```python
from build123d import *

# Parameters (mm, degrees)
SKETCH_1_R          = 7
EXTRUDE_1_DEPTH     = 25
CUT_EXTRUDE_START   = 25
SKETCH_2_R          = 2.5
CUT_EXTRUDE_1_DEPTH = 10
SKETCH_3_R          = 4
CUT_EXTRUDE_2_DEPTH = 15
FILLET_1_R          = 0.25
CHAMFER_1_SIZE      = 0.3


with BuildPart() as part:
    # 草图1 → 凸台-拉伸1 (new body)
    with BuildSketch(Plane(origin=(0, 0, 0), x_dir=(1, 0, 0), z_dir=(0, 1, 0))):
        with Locations(Location((0, 0, 0), (0, 0, 270))):
            Circle(SKETCH_1_R)
    extrude(amount=EXTRUDE_1_DEPTH)

    # 草图2 → 切除-拉伸1 (cut)
    with BuildSketch(Plane(origin=(0, 0, 0), x_dir=(1, 0, 0), z_dir=(0, 1, 0)).offset(CUT_EXTRUDE_START)):
        with Locations(Location((0, 0, 0), (0, 0, 270))):
            Circle(SKETCH_2_R)
    extrude(amount=-CUT_EXTRUDE_1_DEPTH, mode=Mode.SUBTRACT)

    # 草图3 → 切除-拉伸2 (cut)
    with BuildSketch(Plane(origin=(0, 0, 0), x_dir=(1, 0, 0), z_dir=(0, 1, 0))):
        with Locations(Location((0, 0, 0), (0, 0, 270))):
            Circle(SKETCH_3_R)
    extrude(amount=CUT_EXTRUDE_2_DEPTH, mode=Mode.SUBTRACT)

    # 圆角1
    fillet_1_edges = [part.edges().sort_by_distance(p)[0] for p in [
        (0, 0, -7),
        (0, 25, -7),
    ]]
    fillet(fillet_1_edges, radius=FILLET_1_R)

    # 倒角1
    chamfer_1_edges = [part.edges().sort_by_distance(p)[0] for p in [
        (0, 0, -4),
        (0, 25, -2.5),
    ]]
    chamfer(chamfer_1_edges, length=CHAMFER_1_SIZE)


solid = part.part
```
Part model, mm, in its own coordinate system. A direction names the side the tool comes from. Coordinates: 2 decimals unless noted, no trailing zeros. Loops run counter-clockwise (first coordinate to the right, second up) from the corner with the lowest first, then second, coordinate; pieces in that order, holes last. Notation, with made-up numbers: (-19, 8) - (-14, 8) arc R7 cw to (-14, 15) - close; hole circle Ø8 at (-5, 46.25). An arc over 180 degrees is marked (long way). Write item = value, one per line. Start each with the question number.
Item 1: Cut at A-A, the plane z = 0. Give the cut face in (x, y), and give its area (3 significant figures).
Item 2: Cut at B-B, the plane x = 0. Give the cut face in (y, z), and give its area (3 significant figures).
Item 3: Mould opens along X. For faces 1 (the cylindrical face through (-6.834, 12.328, -1.517)), 2 (the flat face through (-1.4, 0, 4.4)), 3 (the cylindrical face through (-3.905, 7.547, -0.867)) say: released by +X, released by -X, zero draft, split by the parting line, or undercut.
Item 4: Cut at D-D, the plane y = 21.75. Give the cut face in (x, z), and give its area (3 significant figures).
Item 5: Wall check: L1, parallel to X at y = 8.25, z = 0; L2, parallel to X at y = 18, z = 0; L3, parallel to Z at x = -0.75, y = 8.75. Give the ranges that are in metal, low to high. Write a range as from..to.
Item 6: Flat gauge pins, fed straight in: pin 1 Ø1 at (x, z) = (3, -5.5) entering from -Y; pin 2 Ø3 at (y, z) = (11, -5) entering from -X; pin 3 Ø2 at (x, y) = (2, 20) entering from -Z; pin 4 Ø4.5 at (x, z) = (0, 0) entering from -Y. Where does each tip first touch, or does it go through?
Item 7: 3-axis set-ups, long thin cutter, end or side, ignore diameter. For faces 4 (the flat face through (2, 15, 2)), 5 (the flat face through (0, 25, 3)): which of +Z, -Z, +X, -X, +Y, -Y reach the whole face in a straight line?
Item 8: Cut at C-C, the plane y = 4.25. Give the cut face in (x, z).
The answers:
q1.outline = (-7, 0.25) arc R0.25 ccw to (-6.75, 0) - (-4.3, 0) - (-4, 0.3) - (-4, 15) - (-2.5, 15) - (-2.5, 24.7) - (-2.8, 25) - (-6.75, 25) arc R0.25 ccw to (-7, 24.75) - close; (2.5, 15) - (4, 15) - (4, 0.3) - (4.3, 0) - (6.75, 0) arc R0.25 ccw to (7, 0.25) - (7, 24.75) arc R0.25 ccw to (6.75, 25) - (2.8, 25) - (2.5, 24.7) - close
q1.area = 180 mm2
q2.outline = (0, -6.75) arc R0.25 ccw to (0.25, -7) - (24.75, -7) arc R0.25 ccw to (25, -6.75) - (25, -2.8) - (24.7, -2.5) - (15, -2.5) - (15, -4) - (0.3, -4) - (0, -4.3) - close; (0, 4.3) - (0.3, 4) - (15, 4) - (15, 2.5) - (24.7, 2.5) - (25, 2.8) - (25, 6.75) arc R0.25 ccw to (24.75, 7) - (0.25, 7) arc R0.25 ccw to (0, 6.75) - close
q2.area = 180 mm2
q3.face_1 = split by the parting line
q3.face_2 = zero draft
q3.face_3 = undercut
q4.outline = circle Ø14 at (0, 0); hole circle Ø5 at (0, 0)
q4.area = 134 mm2
q5.L1 = -7..-4, 4..7
q5.L2 = -7..-2.5, 2.5..7
q5.L3 = -6.96..-3.93, 3.93..6.96
q6.pin_1 = 0
q6.pin_2 = -6.06
q6.pin_3 = -6.93
q6.pin_4 = through
q7.face_4 = -Y
q7.face_5 = +Z, -Z, +X, -X, +Y
q8.outline = circle Ø14 at (0, 0); hole circle Ø8 at (0, 0)
